from build123d import *

# Parameters (mm, degrees)
SKETCH1_R                 = 20
BOSS_EXTRUDE1_DEPTH       = 25
BOSS_EXTRUDE2_START       = 100
SKETCH2_R                 = 20
BOSS_EXTRUDE2_DEPTH       = 100
BOSS_EXTRUDE4_START       = -100
SKETCH6_R                 = 20
BOSS_EXTRUDE4_DEPTH       = 100
SKETCH7_R                 = 25
CUT_EXTRUDE2_DEPTH        = 40
SKETCH8_R                 = 25
SKETCH8_R_2               = 22.5
BOSS_EXTRUDE7_DEPTH       = 40
SKETCH9_R                 = 25
BOSS_EXTRUDE8_DEPTH       = 2
BOSS_EXTRUDE10_DEPTH      = 38
CUT_EXTRUDE3_DEPTH        = 25
SKETCH12_R                = 25
CUT_EXTRUDE4_DEPTH        = 75
BOSS_EXTRUDE11_START      = 50
SKETCH14_R                = 20
BOSS_EXTRUDE11_DEPTH      = 50
BOSS_EXTRUDE12_DEPTH      = 10
BOSS_EXTRUDE12_DEPTH_BACK = 50
SKETCH13_R                = 37.5
SKETCH17_R                = 32.5
CUT_EXTRUDE5_DEPTH        = 50
BOSS_EXTRUDE13_START      = 2
SKETCH18_R                = 37.5
SKETCH18_R_2              = 32.5
BOSS_EXTRUDE13_DEPTH      = 2
SKETCH21_R                = 37.5
SKETCH21_R_2              = 32.5
CUT_EXTRUDE6_DEPTH        = 2
SKETCH22_R                = 1.5
CUT_EXTRUDE7_DEPTH        = 10


with BuildPart() as part:
    # Sketch1 → Boss-Extrude1 (new body)
    with BuildSketch(Plane(origin=(0, 0, 0), x_dir=(1, 0, 0), z_dir=(0, 1, 0))):
        with Locations(Location((0, 0, 0), (0, 0, 270))):
            Circle(SKETCH1_R)
        Polygon((14.43375673, 0), (7.216878365, 12.5), (-7.216878365, 12.5), (-14.43375673, 0), (-7.216878365, -12.5), (7.216878365, -12.5), align=None, mode=Mode.SUBTRACT)
    extrude(amount=BOSS_EXTRUDE1_DEPTH)

    # Sketch2 → Boss-Extrude2 (add)
    with BuildSketch(Plane.XZ.offset(BOSS_EXTRUDE2_START)):
        with Locations(Location((0, 0, 0), (0, 0, 270))):
            Circle(SKETCH2_R)
    extrude(amount=-BOSS_EXTRUDE2_DEPTH)

    # Sketch6 → Boss-Extrude4 (add)
    with BuildSketch(Plane(origin=(0, 25, 0), x_dir=(1, 0, 0), z_dir=(0, 1, 0)).offset(BOSS_EXTRUDE4_START)):
        with Locations(Location((0, 0, 0), (0, 0, 90))):
            Circle(SKETCH6_R)
    extrude(amount=BOSS_EXTRUDE4_DEPTH)

    # Sketch7 → Cut-Extrude2 (cut)
    with BuildSketch(Plane(origin=(20, 0, 0), x_dir=(0, 0, -1), z_dir=(1, 0, 0))):
        with Locations((0, 39.286563349)):
            Circle(SKETCH7_R)
    extrude(amount=-CUT_EXTRUDE2_DEPTH, mode=Mode.SUBTRACT)

    # Sketch8 → Boss-Extrude7 (add)
    with BuildSketch(Plane(origin=(20, 0, 0), x_dir=(0, 0, -1), z_dir=(1, 0, 0))):
        with Locations((0, 39.252781264)):
            Circle(SKETCH8_R)
        with Locations((0, 39.252781264)):
            Circle(SKETCH8_R_2, mode=Mode.SUBTRACT)
    extrude(amount=-BOSS_EXTRUDE7_DEPTH)

    # Sketch9 → Boss-Extrude8 (add)
    with BuildSketch(Plane(origin=(20, 0, 0), x_dir=(0, 0, -1), z_dir=(1, 0, 0))):
        with Locations((0, 39.252781264)):
            Circle(SKETCH9_R)
    extrude(amount=-BOSS_EXTRUDE8_DEPTH)

    # Sketch10 → Boss-Extrude10 (add)
    with BuildSketch(Plane.ZY.offset(-18)):
        with BuildLine():
            Line((-15.081099266, 22.555163323), (15.081099266, 22.555163323))
            ThreePointArc((15.081099266, 22.555163323), (0, 16.752781264), (-15.081099266, 22.555163323))
        make_face()
    extrude(amount=BOSS_EXTRUDE10_DEPTH)

    # Sketch11 → Cut-Extrude3 (cut)
    with BuildSketch(Plane.XZ.offset(100)):
        Polygon((12.5, 7.216878365), (0, 14.43375673), (0, 0), (12.5, 0), align=None)
        Polygon((0, 0), (0, 14.43375673), (-12.5, 7.216878365), (-12.5, -7.216878365), (0, -14.43375673), (12.5, -7.216878365), (12.5, 0), align=None)
    extrude(amount=-CUT_EXTRUDE3_DEPTH, mode=Mode.SUBTRACT)

    # Sketch12 → Cut-Extrude4 (cut)
    with BuildSketch(Plane(origin=(20, 0, 0), x_dir=(0, 0, -1), z_dir=(1, 0, 0))):
        with Locations((0, 39.252781264)):
            Circle(SKETCH12_R)
    extrude(amount=-CUT_EXTRUDE4_DEPTH, mode=Mode.SUBTRACT)

    # Sketch14 → Boss-Extrude11 (add)
    with BuildSketch(Plane.XZ.offset(100).offset(BOSS_EXTRUDE11_START)):
        with Locations(Location((0, 0, 0), (0, 0, 270))):
            Circle(SKETCH14_R)
        Polygon((0, -14.43375673), (12.5, -7.216878365), (12.5, 7.216878365), (0, 14.43375673), (-12.5, 7.216878365), (-12.5, -7.216878365), align=None, mode=Mode.SUBTRACT)
    extrude(amount=-BOSS_EXTRUDE11_DEPTH)

    # Sketch13 → Boss-Extrude12 (add, two sides: drawn at the far end of the back side and taken through both)
    with BuildSketch(Plane(origin=(20, 0, 0), x_dir=(0, 0, -1), z_dir=(1, 0, 0)).offset(-BOSS_EXTRUDE12_DEPTH_BACK)):
        with Locations((0, 39.33472939)):
            Circle(SKETCH13_R)
    extrude(amount=BOSS_EXTRUDE12_DEPTH + BOSS_EXTRUDE12_DEPTH_BACK)

    # Sketch17 → Cut-Extrude5 (cut)
    with BuildSketch(Plane(origin=(30, 0, 0), x_dir=(0, 0, -1), z_dir=(1, 0, 0))):
        with Locations((0, 39.33472939)):
            Circle(SKETCH17_R)
    extrude(amount=-CUT_EXTRUDE5_DEPTH, mode=Mode.SUBTRACT)

    # Sketch18 → Boss-Extrude13 (add)
    with BuildSketch(Plane(origin=(30, 0, 0), x_dir=(0, 0, -1), z_dir=(1, 0, 0)).offset(BOSS_EXTRUDE13_START)):
        with Locations((0, 39.33472939)):
            Circle(SKETCH18_R)
        with Locations((0, 39.33472939)):
            Circle(SKETCH18_R_2, mode=Mode.SUBTRACT)
    extrude(amount=-BOSS_EXTRUDE13_DEPTH)

    # Sketch21 → Cut-Extrude6 (cut)
    with BuildSketch(Plane(origin=(32, 0, 0), x_dir=(0, 0, -1), z_dir=(1, 0, 0))):
        with Locations((0, 39.33472939)):
            Circle(SKETCH21_R)
        with Locations((0, 39.33472939)):
            Circle(SKETCH21_R_2, mode=Mode.SUBTRACT)
    extrude(amount=-CUT_EXTRUDE6_DEPTH, mode=Mode.SUBTRACT)

    # Sketch22 → Cut-Extrude7 (cut)
    with BuildSketch(Plane(origin=(30, 0, 0), x_dir=(0, 0, -1), z_dir=(1, 0, 0))):
        with Locations((0, 74.33472939)):
            Circle(SKETCH22_R)
        with Locations((0, 4.33472939)):
            Circle(SKETCH22_R)
    extrude(amount=-CUT_EXTRUDE7_DEPTH, mode=Mode.SUBTRACT)


solid = part.part
Geometry: final body of the model. Coordinates: model frame, mm. A direction names the side the tool comes from. Give positions to 0.01 mm unless a question says otherwise; leave off trailing zeros. Order: outer loops, then holes, each group sorted by start corner. A loop starts at its lowest first (then second) coordinate and runs counter-clockwise, first axis right, second up. Notation, with made-up numbers: (40, 80) -> (58, 80) arc R9 cw to (58, 89) -> close; hole circle Ø1 at (32.5, 31). An arc over 180 degrees is marked (long way). Put each result on its own line as item: value.
Q1. Section A-A, the plane y = -101. Return loops of the section in (x, z).
Here are the results:
outline: circle Ø40 at (0, 0); hole (-12.5, -7.22) -> (0, -14.43) -> (12.5, -7.22) -> (12.5, 7.22) -> (0, 14.43) -> (-12.5, 7.22) -> close
Q2. Section B-B, the plane x = 6. Return loops of the section in (y, z).
Here are the results:
outline: (-150, -19.08) -> (7.05, -19.08) arc R37.5 ccw (long way) to (7.05, 19.08) -> (-150, 19.08) -> (-150, 10.97) -> (-75, 10.97) -> (-75, -10.97) -> (-150, -10.97) -> close; hole circle Ø65 at (39.33, 0)
Q3. Section D-D, the plane x = -23.5. Return loops of the section in (y, z), then the cut area to 3 significant figures.
Here are the results:
outline: circle Ø75 at (39.33, 0)
area: 4,420 mm^2
Q4. Reachability of faces 1 (the face through (12.5, -113, 0)), 2 (the face through (30, 73, 3)), 3 (the face through (5.35, 7.61, 7.05)) from +Z, -Z, +X, -X, +Y, -Y: full face, straight path, thin tool, end or side. Return the list, or none.
Here are the results:
face 1: -Y
face 2: +Z, -Z, +X, +Y, -Y
face 3: +X
Q5. Draft query along Y for faces 4 (the face through (6.337, -113.025, 10.775)), 5 (the face through (-20, 40, 0)), 6 (the face through (0, -75, 0)). Return one class per face: released by +Y, released by -Y, zero draft, split by the parting line, or undercut.
Here are the results:
face 4: zero draft
face 5: undercut
face 6: released by -Y
Q6. Pin query (flat end, axial travel): pin 1 (10 mm diameter, centred on y = -119, z = -12.5, fed in from -X); pin 2 (8 mm diameter, centred on x = 16.5, y = -109, fed in from +Z); pin 3 (8 mm diameter, centred on x = 13.5, z = 6.5, fed in from +Y). Return the tip coordinate at first contact, or that it passes through.
Here are the results:
pin 1: stops at x = -18.54
pin 2: stops at z = 15.61
pin 3: stops at y = 76.75
Q7. Section C-C, the plane y = 23. Return loops of the section in (x, z), then the cut area to 3 significant figures.
Here are the results:
outline: (-30, -33.76) -> (30, -33.76) -> (30, -28.1) -> (-20, -28.1) -> (-20, 28.1) -> (30, 28.1) -> (30, 33.76) -> (-30, 33.76) -> close
area: 1,240 mm^2
Q8. Material intervals for L1, parallel to Y at x = 22, z = 0; L2, parallel to Y at x = 18.5, z = 0; L3, parallel to Y at x = -15, z = -1, sorted ascending.
Here are the results:
L1: y = 1.83 to 2.83, 5.83 to 6.83, 71.83 to 72.83, 75.83 to 76.83
L2: y = -150 to 6.83, 71.83 to 76.83
L3: y = -150 to 6.85, 71.82 to 76.82
